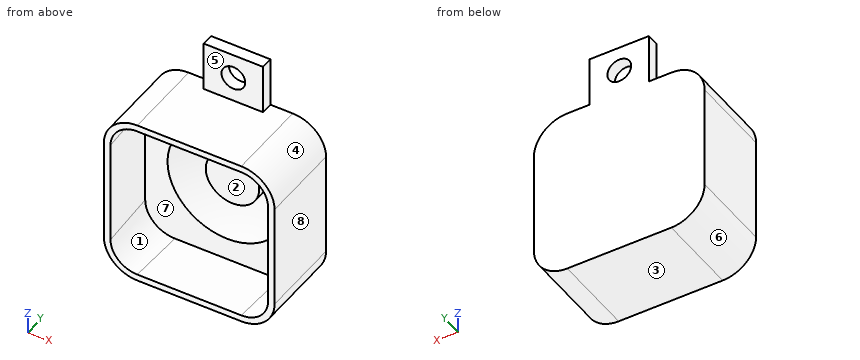
from build123d import *

# Parameters (mm, degrees)
F0_R      = 20
F0_R_2    = 9
F2_DEPTH  = 20.5
F3_SIZE2  = 20.49999
F3_SIZE   = 0.99999
F5_DEPTH  = 3.5
F7_DEPTH  = 28
F9_W      = 20
F9_H      = 8.2
F9_H_2    = 16.8
F9_R      = 4
F10_DEPTH = 4


# Not quite as in the source:
# - a fillet or chamfer is up to 0.001 mm smaller than in the source, because OpenCascade refuses the exact size
# - a feature names something its author has since deleted; it is built from what else it names


with BuildPart() as f2:
    # F0 (on Front) → F2 (new body)
    with BuildSketch(Plane.XZ):
        with BuildLine():
            Line((-17.5, -27.5), (17.5, -27.5))
            ThreePointArc((17.5, -27.5), (24.5710678119, -24.5710678119), (27.5, -17.5))
            Line((27.5, -17.5), (27.5, 17.5))
            ThreePointArc((27.5, 17.5), (24.5710678119, 24.5710678119), (17.5, 27.5))
            Line((17.5, 27.5), (-17.5, 27.5))
            ThreePointArc((-17.5, 27.5), (-24.5710678119, 24.5710678119), (-27.5, 17.5))
            Line((-27.5, 17.5), (-27.5, -17.5))
            ThreePointArc((-27.5, -17.5), (-24.5710678119, -24.5710678119), (-17.5, -27.5))
        make_face()
        with BuildLine():
            ThreePointArc((17.5, 26.5), (23.8639610307, 23.8639610307), (26.5, 17.5))
            Line((26.5, 17.5), (26.5, -17.5))
            ThreePointArc((26.5, -17.5), (23.8639610307, -23.8639610307), (17.5, -26.5))
            Line((17.5, -26.5), (-17.5, -26.5))
            ThreePointArc((-17.5, -26.5), (-23.8639610307, -23.8639610307), (-26.5, -17.5))
            Line((-26.5, -17.5), (-26.5, 17.5))
            ThreePointArc((-26.5, 17.5), (-23.8639610307, 23.8639610307), (-17.5, 26.5))
            Line((-17.5, 26.5), (17.5, 26.5))
        make_face(mode=Mode.SUBTRACT)
        with BuildLine():
            Line((26.5, -17.5), (26.5, 17.5))
            ThreePointArc((26.5, 17.5), (23.8639610307, 23.8639610307), (17.5, 26.5))
            Line((17.5, 26.5), (-17.5, 26.5))
            ThreePointArc((-17.5, 26.5), (-23.8639610307, 23.8639610307), (-26.5, 17.5))
            Line((-26.5, 17.5), (-26.5, -17.5))
            ThreePointArc((-26.5, -17.5), (-23.8639610307, -23.8639610307), (-17.5, -26.5))
            Line((-17.5, -26.5), (17.5, -26.5))
            ThreePointArc((17.5, -26.5), (23.8639610307, -23.8639610307), (26.5, -17.5))
        make_face()
        with BuildLine():
            ThreePointArc((17.5, 25.5), (23.1568542495, 23.1568542495), (25.5, 17.5))
            Line((25.5, 17.5), (25.5, -17.5))
            ThreePointArc((25.5, -17.5), (23.1568542495, -23.1568542495), (17.5, -25.5))
            Line((17.5, -25.5), (-17.5, -25.5))
            ThreePointArc((-17.5, -25.5), (-23.1568542495, -23.1568542495), (-25.5, -17.5))
            Line((-25.5, -17.5), (-25.5, 17.5))
            ThreePointArc((-25.5, 17.5), (-23.1568542495, 23.1568542495), (-17.5, 25.5))
            Line((-17.5, 25.5), (17.5, 25.5))
        make_face(mode=Mode.SUBTRACT)
        with BuildLine():
            Line((25.5, -17.5), (25.5, 17.5))
            ThreePointArc((25.5, 17.5), (23.1568542495, 23.1568542495), (17.5, 25.5))
            Line((17.5, 25.5), (-17.5, 25.5))
            ThreePointArc((-17.5, 25.5), (-23.1568542495, 23.1568542495), (-25.5, 17.5))
            Line((-25.5, 17.5), (-25.5, -17.5))
            ThreePointArc((-25.5, -17.5), (-23.1568542495, -23.1568542495), (-17.5, -25.5))
            Line((-17.5, -25.5), (17.5, -25.5))
            ThreePointArc((17.5, -25.5), (23.1568542495, -23.1568542495), (25.5, -17.5))
        make_face()
        Circle(F0_R, mode=Mode.SUBTRACT)
        Circle(F0_R)
        Circle(F0_R_2, mode=Mode.SUBTRACT)
        Circle(F0_R_2)
    extrude(amount=F2_DEPTH)

    # F3 (size 1 and 20.5 in the source; OpenCascade refuses exactly that, so slightly less here)
    f3_edges = [f2.edges().sort_by_distance(p)[0] for p in [
        (0, -20.5, -27.5),
        (24.571068, -20.5, -24.571068),
        (27.5, -20.5, 0),
        (24.571068, -20.5, 24.571068),
        (0, -20.5, 27.5),
        (-24.571068, -20.5, 24.571068),
        (-27.5, -20.5, 0),
        (-24.571068, -20.5, -24.571068),
    ]]
    f3_side = f2.faces().sort_by_distance((0, -20.5, 0))[0]
    chamfer(f3_edges, length=F3_SIZE, length2=F3_SIZE2, reference=f3_side)

    # F1 (on Top) → F4 (revolve)
    with BuildSketch(Plane.XY):
        with BuildLine():
            Line((9, 0), (20, 0))
            ThreePointArc((20, 0), (14.8597611017, 3.8588264798), (9, 6.5))
            Line((9, 6.5), (0, 6.5))
            Line((0, 6.5), (0, 0))
            Line((0, 0), (9, 0))
        make_face()
    revolve(axis=Axis((0, 3.25, 0), (0, 1, 0)))

    # F5 (cut): a face of the model
    f5_faces = [f2.faces().sort_by_distance(p)[0] for p in [
        (0, 6.5, 0),
    ]]
    extrude(f5_faces, amount=-F5_DEPTH, mode=Mode.SUBTRACT)


with BuildPart() as f7:
    # F6 (on face) → F7 (new body)
    with BuildSketch(Plane.XZ.offset(20.5)):
        with BuildLine():
            Line((-28.7, 17.5), (-28.7, -17.5))
            ThreePointArc((-28.7, -17.5), (-25.4195959493, -25.4195959493), (-17.5, -28.7))
            Line((-17.5, -28.7), (17.5, -28.7))
            ThreePointArc((17.5, -28.7), (25.4195959493, -25.4195959493), (28.7, -17.5))
            Line((28.7, -17.5), (28.7, 17.5))
            ThreePointArc((28.7, 17.5), (25.4195959493, 25.4195959493), (17.5, 28.7))
            Line((17.5, 28.7), (-17.5, 28.7))
            ThreePointArc((-17.5, 28.7), (-25.4195959493, 25.4195959493), (-28.7, 17.5))
        make_face()
        with BuildLine():
            Line((17.5, -26.50001), (-17.5, -26.50001))
            ThreePointArc((-17.5, -26.50001), (-23.8639681017, -23.8639681017), (-26.50001, -17.5))
            Line((-26.50001, -17.5), (-26.50001, 17.5))
            ThreePointArc((-26.50001, 17.5), (-23.8639681017, 23.8639681017), (-17.5, 26.50001))
            Line((-17.5, 26.50001), (17.5, 26.50001))
            ThreePointArc((17.5, 26.50001), (23.8639681017, 23.8639681017), (26.50001, 17.5))
            Line((26.50001, 17.5), (26.50001, -17.5))
            ThreePointArc((26.50001, -17.5), (23.8639681017, -23.8639681017), (17.5, -26.50001))
        make_face(mode=Mode.SUBTRACT)
        with BuildLine():
            ThreePointArc((-26.50001, -17.5), (-23.8639681017, -23.8639681017), (-17.5, -26.50001))
            Line((-17.5, -26.50001), (17.5, -26.50001))
            ThreePointArc((17.5, -26.50001), (23.8639681017, -23.8639681017), (26.50001, -17.5))
            Line((26.50001, -17.5), (26.50001, 17.5))
            ThreePointArc((26.50001, 17.5), (23.8639681017, 23.8639681017), (17.5, 26.50001))
            Line((17.5, 26.50001), (-17.5, 26.50001))
            ThreePointArc((-17.5, 26.50001), (-23.8639681017, 23.8639681017), (-26.50001, 17.5))
            Line((-26.50001, 17.5), (-26.50001, -17.5))
        make_face()
    extrude(amount=-F7_DEPTH)

    # F8: cut F2
    add(f2.part, mode=Mode.SUBTRACT)

    # F9 (on face) → F10 (join)
    with BuildSketch(Plane(origin=(0, 7.5, 0), x_dir=(-1, 0, 0), z_dir=(0, 1, 0))):
        with Locations((0, 24.6)):
            Rectangle(F9_W, F9_H)
        with Locations((0, 37.1)):
            Rectangle(F9_W, F9_H_2)
        with Locations((0, 37.1)):
            Circle(F9_R, mode=Mode.SUBTRACT)
    extrude(amount=-F10_DEPTH)


solid = f7.part
Input: part model. Units: mm. Frame: model coordinates. Face numbers are marked on the shaded views. A direction names the side the tool comes from. Coordinates: 2 decimals unless noted, no trailing zeros. Order: outer loops, then holes, each group sorted by start corner. A loop starts at its lowest first (then second) coordinate and runs counter-clockwise, first axis right, second up.
1. Ray query, line 1 along Z through (x, y) = (0, 5.4); line 2 along Z through (x, y) = (0, 5.15); line 3 along Y through (x, z) = (-25.5, -11). Return the intervals inside material, ascending.
Checked values:
line 1: z = -28.7 to -11.87, -9 to 9, 11.87 to 33.1, 41.1 to 45.5
line 2: z = -28.7 to -12.42, -9 to 9, 12.42 to 33.1, 41.1 to 45.5
line 3: y = 0 to 7.5
2. Draft query along X for the marked faces 6, 7 and 8. Return one class per face: +X half, -X half, draft (parallel to the pull), parting line (faces both ways), or undercut.
Checked values:
face 6: -X half
face 7: undercut
face 8: +X half
3. Cut plane A-A, the plane z = 37.1. Return loops of the section in (x, y), plus the area to 3 significant figures.
Checked values:
outline: (-10, 3.5) - (-4, 3.5) - (-4, 7.5) - (-10, 7.5) - close; (4, 3.5) - (10, 3.5) - (10, 7.5) - (4, 7.5) - close
area: 48.0 mm2
4. Cut plane C-C, the plane y = -1.25. Return loops of the section in (x, z).
Checked values:
outline: (-28.7, -17.5) arc R11.2 ccw to (-17.5, -28.7) - (17.5, -28.7) arc R11.2 ccw to (28.7, -17.5) - (28.7, 17.5) arc R11.2 ccw to (17.5, 28.7) - (-17.5, 28.7) arc R11.2 ccw to (-28.7, 17.5) - close; hole (-27.44, -17.5) arc R9.94 ccw to (-17.5, -27.44) - (17.5, -27.44) arc R9.94 ccw to (27.44, -17.5) - (27.44, 17.5) arc R9.94 ccw to (17.5, 27.44) - (-17.5, 27.44) arc R9.94 ccw to (-27.44, 17.5) - close
5. Contact query for flat-ended pins moving along their axis: P1, Ø2, axis at y = 4.5, z = 40, coming from the +X side; P2, Ø8.5, axis at x = 3.5, z = 37, coming from the -Y side; P3, Ø1.2, axis at y = 6.5, z = 33.5, coming from the -X side; P4, Ø6.5, axis at x = 0, z = 37.1, coming from the -Y side. Output: stop coordinate, or through.
Checked values:
P1: stops at x = 10
P2: stops at y = 3.5
P3: stops at x = -10
P4: passes through
6. Access query for the marked faces 1, 2, 3, 4 and 5. Directions: +Z, -Z, +X, -X, +Y, -Y. A direction counts if a zero-diameter tool reaches every point of the face in a straight line with its end or side. Return the directions, or none.
Checked values:
face 1: none
face 2: -Y
face 3: -Z, +X, -X, +Y, -Y
face 4: +Z, +X, +Y, -Y
face 5: +Z, +X, -X, -Y
